```python
from build123d import *

# Parameters (mm, degrees)
BASE_EXTRUSION_DEPTH    = 17
ENL_V_MAT_EXTRU_1_DEPTH = 17
ESQUISSE3_R             = 11.5
BOSS_EXTRU_1_DEPTH      = 3
ESQUISSE4_R             = 10
ENL_V_MAT_EXTRU_2_DEPTH = 3
ENL_V_MAT_EXTRU_3_DEPTH = 3


with BuildPart() as part:
    # Esquisse1 → Base-Extrusion (new body)
    with BuildSketch(Plane.XY):
        with BuildLine():
            Line((-16, -10.124371965), (-7.331240844, -10.124371965))
            ThreePointArc((-7.331240844, -10.124371965), (0, -12.5), (7.331240844, -10.124371965))
            Line((7.331240844, -10.124371965), (16, -10.124371965))
            ThreePointArc((16, -10.124371965), (19.535533906, -8.659905871), (21, -5.124371965))
            Line((21, -5.124371965), (21, 0.875628035))
            ThreePointArc((21, 0.875628035), (19.535533906, 4.411161941), (16, 5.875628035))
            Line((16, 5.875628035), (12.5, 5.875628035))
            Line((12.5, 5.875628035), (12.5, 15.5))
            ThreePointArc((12.5, 15.5), (0, 20.67766953), (-12.5, 15.5))
            Line((-12.5, 15.5), (-12.5, 5.875628035))
            Line((-12.5, 5.875628035), (-16, 5.875628035))
            ThreePointArc((-16, 5.875628035), (-19.535533906, 4.411161941), (-21, 0.875628035))
            Line((-21, 0.875628035), (-21, -5.124371965))
            ThreePointArc((-21, -5.124371965), (-19.535533906, -8.659905871), (-16, -10.124371965))
        make_face()
    extrude(amount=BASE_EXTRUSION_DEPTH)

    # Esquisse2 → Enlèv. mat.-Extru.1 (cut)
    with BuildSketch(Plane.XY.offset(17)):
        with BuildLine():
            Line((-16.5, 3.5), (-15.5, 3.5))
            ThreePointArc((-15.5, 3.5), (-14.085786438, 2.914213562), (-13.5, 1.5))
            Line((-13.5, 1.5), (-13.5, -5.5))
            ThreePointArc((-13.5, -5.5), (-14.085786438, -6.914213562), (-15.5, -7.5))
            Line((-15.5, -7.5), (-16.5, -7.5))
            ThreePointArc((-16.5, -7.5), (-17.914213562, -6.914213562), (-18.5, -5.5))
            Line((-18.5, -5.5), (-18.5, 1.5))
            ThreePointArc((-18.5, 1.5), (-17.914213562, 2.914213562), (-16.5, 3.5))
        make_face()
        with BuildLine():
            Line((15.5, 3.5), (16.5, 3.5))
            ThreePointArc((16.5, 3.5), (17.914213562, 2.914213562), (18.5, 1.5))
            Line((18.5, 1.5), (18.5, -5.5))
            ThreePointArc((18.5, -5.5), (17.914213562, -6.914213562), (16.5, -7.5))
            Line((16.5, -7.5), (15.5, -7.5))
            ThreePointArc((15.5, -7.5), (14.085786438, -6.914213562), (13.5, -5.5))
            Line((13.5, -5.5), (13.5, 1.5))
            ThreePointArc((13.5, 1.5), (14.085786438, 2.914213562), (15.5, 3.5))
        make_face()
    extrude(amount=-ENL_V_MAT_EXTRU_1_DEPTH, mode=Mode.SUBTRACT)

    # Esquisse3 → Boss.-Extru.1 (add)
    with BuildSketch(Plane.XY.offset(17)):
        Circle(ESQUISSE3_R)
    extrude(amount=BOSS_EXTRU_1_DEPTH)

    # Esquisse4 → Enlèv. mat.-Extru.2 (cut)
    with BuildSketch(Plane.XY.offset(20)):
        Circle(ESQUISSE4_R)
    extrude(amount=-ENL_V_MAT_EXTRU_2_DEPTH, mode=Mode.SUBTRACT)

    # Esquisse5 → Enlèv. mat.-Extru.3 (cut)
    with BuildSketch(Plane.XY.offset(20)):
        with BuildLine():
            Line((-20, 10), (0, 0))
            Line((0, 0), (20, 10))
            ThreePointArc((20, 10), (0, 22.360679775), (-20, 10))
        make_face()
    extrude(amount=-ENL_V_MAT_EXTRU_3_DEPTH, mode=Mode.SUBTRACT)


solid = part.part
```
Input: part model. Units: mm. Frame: model coordinates. A direction names the side the tool comes from. Give positions to 0.01 mm unless a question says otherwise; leave off trailing zeros. Order: outer loops, then holes, each group sorted by start corner. A loop starts at its lowest first (then second) coordinate and runs counter-clockwise, first axis right, second up.
1. Cut plane C-C (x = -17.5). Return loops of the section in (y, z).
Computed:
outline: (-9.89, 0) - (-7.23, 0) - (-7.23, 17) - (-9.89, 17) - close; (3.23, 0) - (5.65, 0) - (5.65, 17) - (3.23, 17) - close
2. Line query: probe 1 along X at (y, z) = (-2, 14.5); probe 2 along X at (y, z) = (0, 19.1); probe 3 along X at (y, z) = (2, 7.5). Output: solid intervals per line, ascending.
Computed:
probe 1: x = -21 to -18.5, -13.5 to 13.5, 18.5 to 21
probe 2: x = -11.5 to -10, 10 to 11.5
probe 3: x = -20.87 to -18.44, -13.56 to 13.56, 18.44 to 20.87
3. Draft query along X for faces 1 (the face through (19.574, 4.372, 8.381)), 2 (the face through (-18.5, -2, 9)), 3 (the face through (-12.5, 11, 8)). Return one class per face: released by +X, released by -X, zero draft, split by the parting line, or undercut.
Computed:
face 1: released by +X
face 2: undercut
face 3: released by -X
4. Cut plane D-D (x = 0). Return loops of the section in (y, z), and give its area (3 significant figures).
Computed:
outline: (-12.5, 0) - (20.68, 0) - (20.68, 17) - (-10, 17) - (-10, 20) - (-11.5, 20) - (-11.5, 17) - (-12.5, 17) - close
area: 569 mm2
5. Pin query (flat end, axial travel): pin 1 Ø0.5 at (x, z) = (16, 5.5) entering from -Y; pin 2 Ø0.5 at (x, z) = (16, 7) entering from +Y; pin 3 Ø12 at (x, z) = (13.5, 9) entering from +Y. Return the tip coordinate at first contact, or that it passes through.
Computed:
pin 1: stops at y = -10.12
pin 2: stops at y = 5.88
pin 3: stops at y = 19.01
6. Cut plane A-A (y = 0). Return loops of the section in (x, z), and give its area (3 significant figures).
Computed:
outline: (-21, 0) - (-18.5, 0) - (-18.5, 17) - (-21, 17) - close; (-13.5, 0) - (13.5, 0) - (13.5, 17) - (11.5, 17) - (11.5, 20) - (10, 20) - (10, 17) - (-10, 17) - (-10, 20) - (-11.5, 20) - (-11.5, 17) - (-13.5, 17) - close; (18.5, 0) - (21, 0) - (21, 17) - (18.5, 17) - close
area: 553 mm2
7. Set-up query: faces 4 (the face through (-10, 5, 19)), 5 (the face through (-14, 5.876, 8)), 6 (the face through (-13.5, -2, 9)). Return all of +Z, -Z, +X, -X, +Y, -Y with unobstructed straight access to the full face (end or side cutting, diameter ignored); none if empty.
Computed:
face 4: +Z, +Y
face 5: +Z, -Z, -X, +Y
face 6: +Z, -Z
8. Cut plane B-B (z = 2.5). State how many separate pieces and enclosed holes the cut face has, and give its area (3 significant figures).
Computed:
separate pieces: 1
enclosed holes: 2
area: 901 mm2
